The listing builds one solid part. Answer for the finished solid, in the listing's coordinates (mm). Face numbers are marked on the shaded views. A direction names the side the tool comes from. Give positions to 0.01 mm unless a question says otherwise; leave off trailing zeros. Write each loop counter-clockwise with the first axis right and the second up, starting at its lowest first coordinate (ties: lowest second). Pieces come first, ordered by that corner, then holes. Notation, with made-up numbers: (40, 42) - (69, 42) arc R29 cw to (69, 62) - close; hole circle Ø2 at (18.25, 67.25). An arc over 180 degrees is marked (long way). Use a Markdown table: item, result. Add a question column.
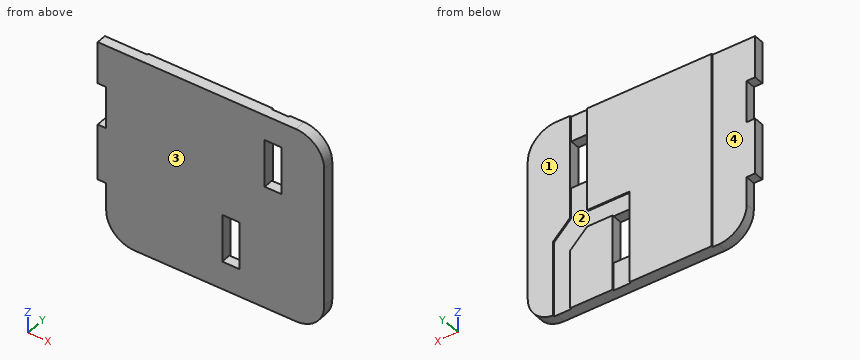
from build123d import *

# Parameters (mm, degrees)
SKETCH1_W           = 0.6
SKETCH1_H           = 1.7
BOSS_EXTRUDE1_DEPTH = 0.4
FILLET1_R           = 1
SKETCH3_W           = 0.6
SKETCH3_H           = 0.9
SKETCH3_H_2         = 1
CUT_EXTRUDE2_DEPTH  = 0.05


with BuildPart() as part:
    # Sketch1 → Boss-Extrude1 (new body)
    with BuildSketch(Plane(origin=(0, 0, 0), x_dir=(1, 0, 0), z_dir=(0, 1, 0))):
        Polygon((0, 0), (8, 0), (8, 7), (0.3, 7), (0.3, 5), (0, 5), (0, 3), (0.3, 3), (0.3, 1.5), (0, 1.5), align=None)
        with Locations((4.7, 5.15)):
            Rectangle(SKETCH1_W, SKETCH1_H, mode=Mode.SUBTRACT)
        with Locations((6.2, 1.75)):
            Rectangle(SKETCH1_W, SKETCH1_H, mode=Mode.SUBTRACT)
    extrude(amount=BOSS_EXTRUDE1_DEPTH)

    # Fillet1
    fillet1_edges = [part.edges().sort_by_distance(p)[0] for p in [
        (0.3, 0.2, -7),
        (8, 0.2, -7),
        (8, 0.2, 0),
    ]]
    fillet(fillet1_edges, radius=FILLET1_R)

    # Sketch3 → Cut-Extrude2 (cut)
    with BuildSketch(Plane(origin=(0, 0.4, 0), x_dir=(1, 0, 0), z_dir=(0, 1, 0))):
        with BuildLine():
            Line((1.5, 0), (1.5, 7))
            Line((1.5, 7), (1.3, 7))
            ThreePointArc((1.3, 7), (0.592893219, 6.707106781), (0.3, 6))
            Line((0.3, 6), (0.3, 5))
            Line((0.3, 5), (0, 5))
            Line((0, 5), (0, 3))
            Line((0, 3), (0.3, 3))
            Line((0.3, 3), (0.3, 1.5))
            Line((0.3, 1.5), (0, 1.5))
            Line((0, 1.5), (0, 0))
            Line((0, 0), (1.5, 0))
        make_face()
        with Locations((6.2, 0.45)):
            Rectangle(SKETCH3_W, SKETCH3_H)
        Polygon((4.4, 4.3), (5, 4.3), (5.9, 4.3), (6.5, 4.9), (6.5, 7), (6.5, 7.268876882), (7.1, 7.268876882), (7.1, 6.994987437), (7.1, 4.3), (6.5, 3.7), (6.5, 2.6), (5.9, 2.6), (5.9, 3.7), (4.4, 3.7), align=None)
        with Locations((4.7, 6.5)):
            Rectangle(SKETCH3_W, SKETCH3_H_2)
    extrude(amount=-CUT_EXTRUDE2_DEPTH, mode=Mode.SUBTRACT)


solid = part.part
1. For a pull along Z with two mould halves and no side action, classify the marked faces 1 and 2 as released by +Z, released by -Z, zero draft, split by the parting line, or undercut.
2. The part is cut by section B-B (x = 6). Give the vertices of the cut face in (y, z), and give its area (4 significant figures).
3. Which of the six approach directions +Z, -Z, +X, -X, +Y, -Y give full straight-line access (tool end or side, diameter ignored) to the marked faces 3 and 4?
4. The part is cut by section C-C (y = 0.15). Give the vertices of the cut face in (x, z).
5. The part is cut by section A-A (z = -5.75). Give the vertices of the cut face in (x, y), and give its area (3 significant figures).
6. Given P1, Ø1, axis at x = 5, z = -6, coming from the -Y side; P2, Ø0.8, axis at x = 0.5, z = -4.5, coming from the +Y side, each flat-ended and moving along its own axis, determine where each tip first touches the part or whether it passes through.
7. The part is cut by section D-D (z = -1.25). Give the vertices of the cut face in (x, y), and give its area (4 significant figures).
8. Consider L1, parallel to X at y = 0.2, z = -1.25; L2, parallel to X at y = 0.25, z = -2.5; L3, parallel to Z at x = 6.25, y = 0.2. Determine where each line is inside the solid, lowest interval first. Write a range as [from, to].
Check values:
| question | item | result |
|---|---|---|
| 1 | face 1 | zero draft |
| 1 | face 2 | undercut |
| 2 | outline | (0, -7) - (0.4, -7) - (0.4, -4.4) - (0.35, -4.4) - (0.35, -2.6) - (0, -2.6) - close; (0, -0.9) - (0.35, -0.9) - (0.35, 0) - (0, 0) - close |
| 2 | area | 1.985 mm2 |
| 3 | face 3 | +Z, -Z, +X, -X, -Y |
| 3 | face 4 | +Z, -Z, -X, +Y |
| 4 | outline | (0, -5) - (0.3, -5) - (0.3, -6) arc R1 ccw to (1.3, -7) - (7, -7) arc R1 ccw to (8, -6) - (8, -1) arc R1 ccw to (7, 0) - (0, 0) - (0, -1.5) - (0.3, -1.5) - (0.3, -3) - (0, -3) - close; hole (4.4, -6) - (5, -6) - (5, -4.3) - (4.4, -4.3) - close; hole (5.9, -2.6) - (6.5, -2.6) - (6.5, -0.9) - (5.9, -0.9) - close |
| 5 | outline | (0.3, 0) - (4.4, 0) - (4.4, 0.4) - (1.5, 0.4) - (1.5, 0.35) - (0.3, 0.35) - close; (5, 0) - (8, 0) - (8, 0.4) - (7.1, 0.4) - (7.1, 0.35) - (6.5, 0.35) - (6.5, 0.4) - (5, 0.4) - close |
| 5 | area | 2.75 mm2 |
| 6 | P1 | stops at y = 0 |
| 6 | P2 | stops at y = 0.35 |
| 7 | outline | (0, 0) - (5.9, 0) - (5.9, 0.4) - (1.5, 0.4) - (1.5, 0.35) - (0, 0.35) - close; (6.5, 0) - (8, 0) - (8, 0.4) - (6.5, 0.4) - close |
| 7 | area | 2.885 mm2 |
| 8 | L1 | x = [0, 5.9], [6.5, 8] |
| 8 | L2 | x = [0.3, 5.9], [6.5, 8] |
| 8 | L3 | z = [-7, -2.6], [-0.9, 0] |
